```python
from build123d import *

# Parameters (mm, degrees)
SKETCH1_W     = 10
SKETCH1_H     = 4
SKETCH1_W_2   = 8
SKETCH1_W_3   = 12
SKETCH1_W_4   = 38
FILLET1_R     = 0.2
CHAMFER1_SIZE = 0.3


with BuildPart() as part:
    # Sketch1 → Revolve1 (revolve)
    with BuildSketch(Plane.XY, mode=Mode.PRIVATE) as revolve1_sk:
        with Locations((5, 2)):
            Rectangle(SKETCH1_W, SKETCH1_H)
        Polygon((10, 4.5), (10, 4), (10, 0), (12, 0), (12, 4), (12, 4.5), align=None)
        with Locations((16, 2)):
            Rectangle(SKETCH1_W_2, SKETCH1_H)
        with Locations((26, 2)):
            Rectangle(SKETCH1_W_3, SKETCH1_H)
        with Locations((36, 2)):
            Rectangle(SKETCH1_W_2, SKETCH1_H)
        Polygon((40, 4), (40, 0), (42, 0), (42, 4), (42, 4.5), (40, 4.5), align=None)
        with Locations((47, 2)):
            Rectangle(SKETCH1_W, SKETCH1_H)
        with Locations((71, 2)):
            Rectangle(SKETCH1_W_4, SKETCH1_H)
    revolve(revolve1_sk.sketch.rotate(Axis((0, 0, 0), (1, 0, 0)), 90), axis=Axis((0, 0, 0), (1, 0, 0)))

    # Fillet1
    fillet1_edges = [part.edges().sort_by_distance(p)[0] for p in [
        (10, 0, -4),
        (12, 0, -4),
        (40, 0, -4),
        (42, 0, -4),
    ]]
    fillet(fillet1_edges, radius=FILLET1_R)

    # Chamfer1
    chamfer1_edges = [part.edges().sort_by_distance(p)[0] for p in [
        (90, 0, -4),
        (0, 0, -4),
    ]]
    chamfer(chamfer1_edges, length=CHAMFER1_SIZE)


solid = part.part
```
Here's how the part is built. I have some questions about the finished solid (model axes, mm). A direction names the side the tool comes from. Coordinates: 2 decimals unless noted, no trailing zeros. Write each loop counter-clockwise with the first axis right and the second up, starting at its lowest first coordinate (ties: lowest second). Pieces come first, ordered by that corner, then holes. Notation, with made-up numbers: (55, 76.25) -> (61, 76.25) arc R26 ccw to (61, 97.25) -> close; hole circle Ø9 at (64, 61.5). An arc over 180 degrees is marked (long way). Use a Markdown table: item, result. Add a question column.
(1) Please list where these lines run through material, in increasing order: line 1 (X direction, y = -2.75, z = 3.5); line 2 (Z direction, x = 81.5, y = -0.25); line 3 (Z direction, x = 85, y = 1.5).
(2) For faces 4 (the cylindrical face through (5.116, 3.905, -0.867)), 5 (the cylindrical face through (65.618, 3.905, -0.867)), 6 (the cylindrical face through (40.99, -3.04, -3.32)), which set-ups out of +Z, -Z, +X, -X, +Y, -Y let a thin tool reach every point of the face, with its end or its side?
(3) I'm going to push flat-ended pins straight in: P1, Ø5, axis at x = 33, z = 1, coming from the +Y side; P2, Ø5, axis at x = 71, y = 0, coming from the -Z side. Where does each tip first touch, or does it pass through?
(4) We'd pull the mould along X, two halves only. Please class faces 1 (the cylindrical face through (10.99, -3.04, -3.32)), 2 (the cylindrical face through (25.807, 3.905, -0.867)), 3 (the flat face through (90, 0, 0)): +X half, -X half, draft (parallel to the pull), parting line (faces both ways), or undercut.
(5) If we section it at C-C, the plane x = 35: Write out the boundary of the cut face in (y, z), and give its area (3 significant figures).
Outcome:
| question | item | result |
|---|---|---|
| 1 | line 1 | x = 10 to 12, 40 to 42 |
| 1 | line 2 | z = -3.99 to 3.99 |
| 1 | line 3 | z = -3.71 to 3.71 |
| 2 | face 4 | -X |
| 2 | face 5 | +X |
| 2 | face 6 | +X, -X |
| 3 | P1 | stops at y = 4 |
| 3 | P2 | stops at z = -4 |
| 4 | face 1 | draft |
| 4 | face 2 | undercut |
| 4 | face 3 | +X half |
| 5 | outline | circle Ø8 at (0, 0) |
| 5 | area | 50.3 mm^2 |
